The figure shows three views and two pictorial views of one solid part (mm, origin at its lowest corner). Answer the questions. A direction names the side the tool comes from. Coordinates: 2 decimals unless noted, no trailing zeros. Loops run counter-clockwise (first coordinate to the right, second up) from the corner with the lowest first, then second, coordinate; pieces in that order, holes last. Notation, with made-up numbers: M 24,86.5 L 69,86.5 A16 ccw 69,91.5 Z; hole C 63.5,-29 d10. An arc over 180 degrees is marked long. One line per item, written item: value. Start each with the question number.
1. The part is cut by section C-C (x = 13.25). Write down the section's boundary in (y, z).
2. Consider probe 1 along X at (y, z) = (5.5, 1); probe 2 along Z at (x, y) = (12, 7); probe 3 along X at (y, z) = (3.25, 6). Determine where each line is inside the solid, lowest interval first.
3. For the marked faces 1, 2 and 3, determine the directions among +Z, -Z, +X, -X, +Y, -Y from which every point of the face is accessible in a straight line to the end or side of a thin tool.
4. The part is cut by section B-B (x = 3.5). Write down the section's boundary in (y, z).
5. Determine the mould class of the marked faces 4, 5 and 6 for opening direction Z: +Z half, -Z half, draft (parallel to the pull), parting line (faces both ways), or undercut.
6. The part is cut by section A-A (z = 6). Write down the section's boundary in (x, y), then the cut area to 3 significant figures.
7. Flat-ended cylindrical pins translate along their axes: pin 1 (1.5 mm diameter, centred on x = 14.5, y = 7.5, fed in from -Z) (1 decimal); pin 2 (2 mm diameter, centred on x = 11.5, z = 8, fed in from -Y); pin 3 (3 mm diameter, centred on x = 10, y = 9.5, fed in from -Z). Find the tip coordinate at first contact, or state that the pin passes through.
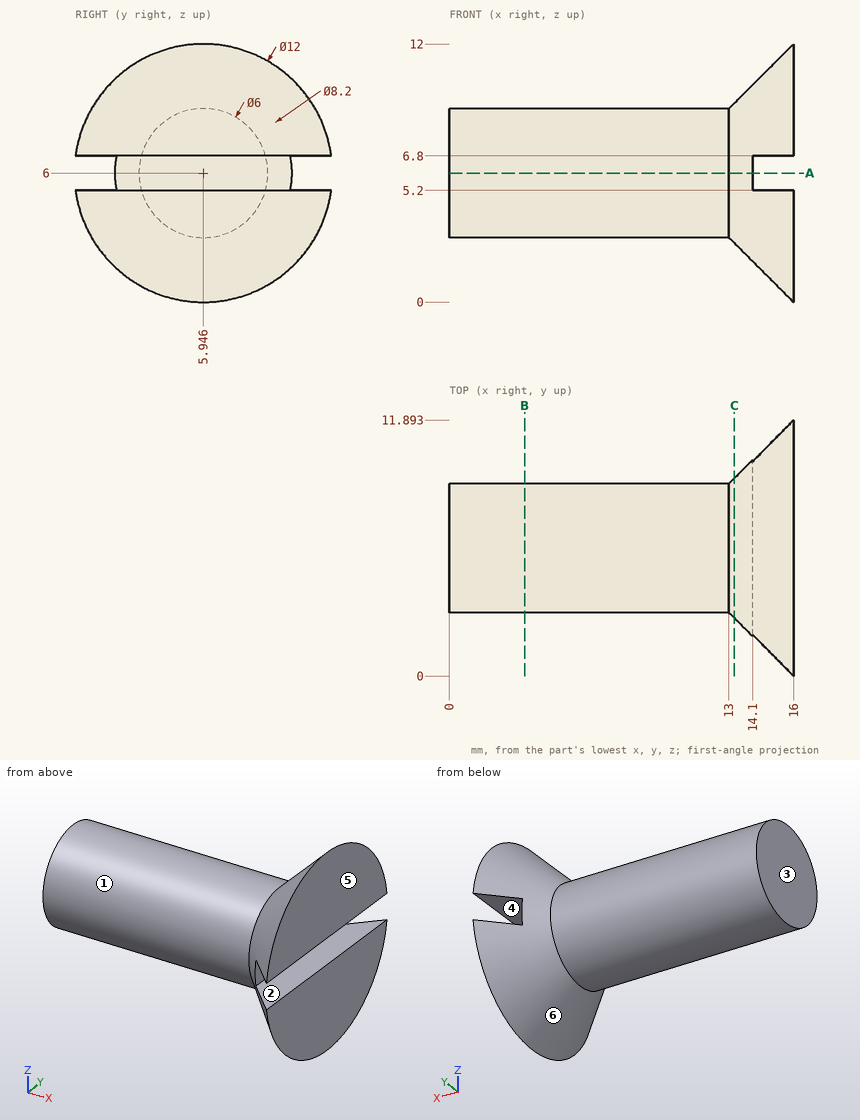
Answer block:
1. outline: C 5.95,6 d6.5
2. probe 1: x = 15.02 to 16
2. probe 2: z = 3.19 to 8.81
2. probe 3: x = 0 to 14.1
3. face 1: -X
3. face 2: +X, +Y, -Y
3. face 3: +Z, -Z, -X, +Y, -Y
4. outline: C 5.95,6 d6
5. face 4: undercut
5. face 5: draft
5. face 6: parting line
6. outline: M 0,2.95 L 13,2.95 L 14.1,1.85 L 14.1,10.05 L 13,8.95 L 0,8.95 Z
6. area: 85.8 mm2
7. pin 1: stops at z = 1
7. pin 2: stops at y = 3.12
7. pin 3: stops at z = 3.81
